from build123d import *

# Parameters (mm, degrees)
SKETCH_W        = 60
SKETCH_H        = 60
SKETCH_W_2      = 54
SKETCH_H_2      = 54
PAD_DEPTH       = 610
SKETCH001_R     = 4.25
POCKET_DEPTH    = 3
SKETCH002_R     = 4.25
POCKET001_DEPTH = 3
FILLET_R        = 3


with BuildPart() as part:
    # Sketch → Pad (new body)
    with BuildSketch(Plane.XZ):
        Rectangle(SKETCH_W, SKETCH_H)
        Rectangle(SKETCH_W_2, SKETCH_H_2, mode=Mode.SUBTRACT)
    extrude(amount=PAD_DEPTH)

    # Sketch001 (on Face1 of Pad) → Pocket (cut)
    with BuildSketch(Plane(origin=(0, 0, 30), x_dir=(-1, 0, 0), z_dir=(0, 0, 1))):
        with Locations((0, 30)):
            Circle(SKETCH001_R)
        with Locations((0, 580)):
            Circle(SKETCH001_R)
    extrude(amount=-POCKET_DEPTH, mode=Mode.SUBTRACT)

    # Sketch002 (on Face8 of Pocket) → Pocket001 (cut)
    with BuildSketch(Plane(origin=(0, 0, -30), x_dir=(1, 0, 0), z_dir=(0, 0, -1))):
        with Locations((0, 30)):
            Circle(SKETCH002_R)
        with Locations((0, 580)):
            Circle(SKETCH002_R)
    extrude(amount=-POCKET001_DEPTH, mode=Mode.SUBTRACT)

    # Fillet
    fillet_edges = [part.edges().sort_by_distance(p)[0] for p in [
        (30, -305, 30),
        (30, -305, -30),
        (-30, -305, -30),
        (-30, -305, 30),
    ]]
    fillet(fillet_edges, radius=FILLET_R)


solid = part.part
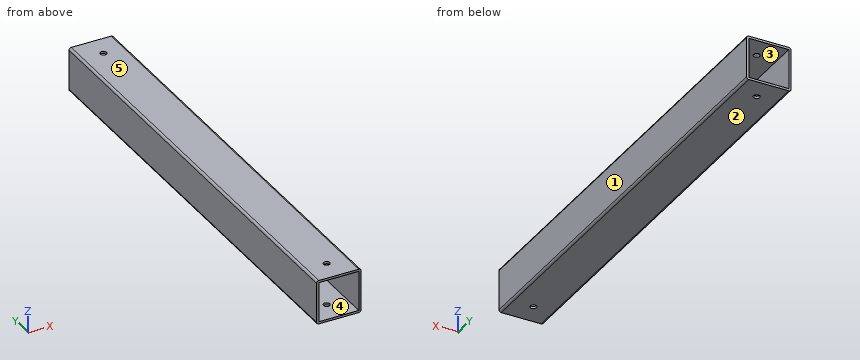
Build history of the part. All positions in model axes, mm. Face numbers are marked on the shaded views. A direction names the side the tool comes from. Round coordinates to 2 decimals unless told otherwise and drop trailing zeros. Write each loop counter-clockwise with the first axis right and the second up, starting at its lowest first coordinate (ties: lowest second). Pieces come first, ordered by that corner, then holes. Notation, with made-up numbers: M 89,-4 L 121,-4 A20 cw 121,13 Z; hole C -34.5,74 d2. An arc over 180 degrees is marked long. Answer as a JSON object with one key per item and string values. Group by question number.
(1) Which spindle directions (+Z, -Z, +X, -X, +Y, -Y) get a long thin tool onto all of the face, cutting with end or side? Do the marked faces 4 and 5. Say none if no direction does.
(2) Cut at B-B (x = -13). Give the cut face in (y, z).
(3) Flat gauge pin, fed straight in: pin 1 (7.5 mm diameter, centred on x = 0, y = -30, fed in from +Z). Where does the tip first touch, or does it go through?
(4) Cut at A-A (z = 4). Give the cut face in (x, y).
(5) Mould opens along X. For the marked faces 1, 2 and 3 say: pulls with the +X half, pulls with the -X half, needs draft (parallel to the pull), parting line crosses it, or undercut.
(6) Drill centre lines: L1, parallel to Y at x = 0, z = -29; L2, parallel to Z at x = 14, y = -492.5. Where is each one in solid material? Low to high.
(7) Cut at C-C (y = -225). Give the cut face in (x, z).
Responses:
{
 "1": {"face 4": "+Y, -Y", "face 5": "+Z, +X, -X, +Y, -Y"},
 "2": {"outline": "M -610,-30 L 0,-30 L 0,-27 L -610,-27 Z; M -610,27 L 0,27 L 0,30 L -610,30 Z"},
 "3": {"pin 1": "passes through"},
 "4": {"outline": "M -30,-610 L -27,-610 L -27,0 L -30,0 Z; M 27,-610 L 30,-610 L 30,0 L 27,0 Z"},
 "5": {"face 1": "pulls with the +X half", "face 2": "needs draft", "face 3": "undercut"},
 "6": {"L1": "y = -610 to -584.25, -575.75 to -34.25, -25.75 to 0", "L2": "z = -30 to -27, 27 to 30"},
 "7": {"outline": "M -30,-27 A3 ccw -27,-30 L 27,-30 A3 ccw 30,-27 L 30,27 A3 ccw 27,30 L -27,30 A3 ccw -30,27 Z; hole M -27,-27 L 27,-27 L 27,27 L -27,27 Z"}
}
